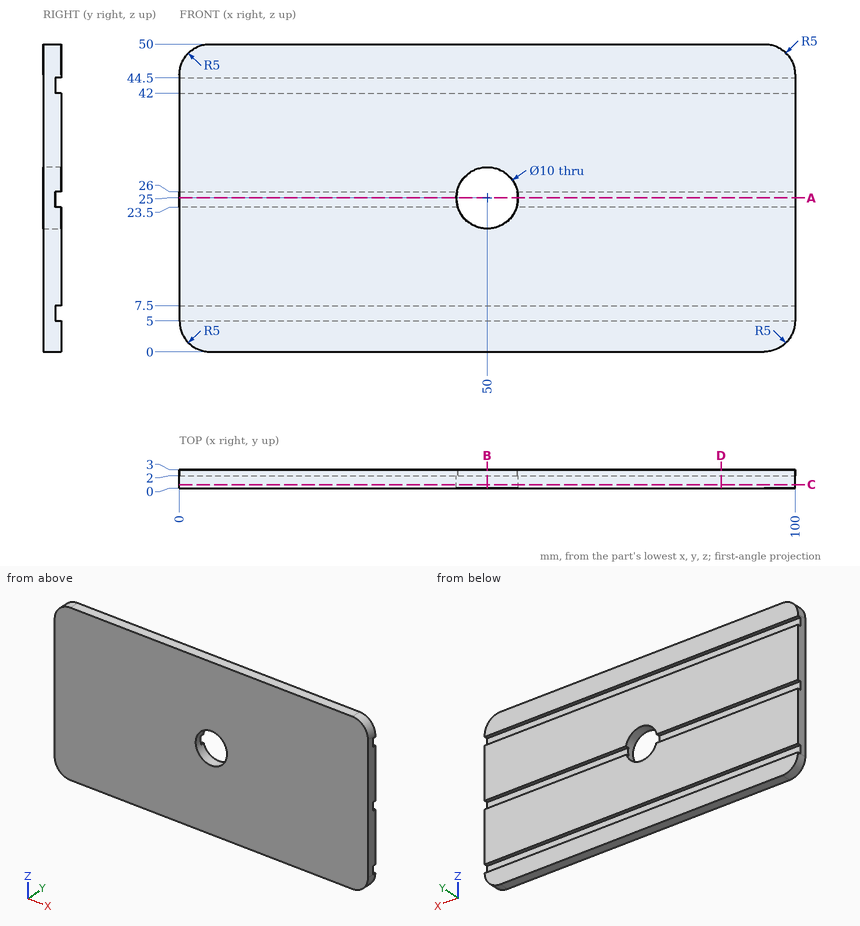
Part print with two shaded views. Sizes in mm from the minimum x, y, z corner. Round coordinates to 2 decimals unless told otherwise and drop trailing zeros. Order: outer loops, then holes, each group sorted by start corner. A loop starts at its lowest first (then second) coordinate and runs counter-clockwise, first axis right, second up. Notation, with made-up numbers: M -34,39 L -5,39 A33 ccw -5,73 Z; hole C 41,2.25 d5. An arc over 180 degrees is marked long. Use CSV: the item, a comma, the result in double quotes. Start each with the question number.
(1) Cut at D-D on x = 88. List the corners of the cut face in (y, z), then the cut area to 4 significant figures.
(2) Flat gauge pin, fed straight in: P1, Ø1.2, axis at x = 30, z = 6.5, coming from the +Y side. Where does the tip first touch, or does it go through?
(3) Drill centre lines: probe 1 along Z at (x, y) = (72, 2.55); probe 2 along Z at (x, y) = (50, 0.75); probe 3 along Z at (x, y) = (47, 2.7). Where is each one in solid material? Low to high.
(4) Cut at C-C on y = 0.6. List the corners of the cut face in (x, z).
(5) Cut at A-A on z = 25. List the corners of the cut face in (x, y).
(6) Cut at B-B on x = 50. List the corners of the cut face in (y, z), then the cut area to 3 significant figures.
Findings:
1,outline,"M 0,0 L 3,0 L 3,5 L 2,5 L 2,7.5 L 3,7.5 L 3,23.5 L 2,23.5 L 2,26 L 3,26 L 3,42 L 2,42 L 2,44.5 L 3,44.5 L 3,50 L 0,50 Z"
1,area,"142.5 mm^2"
2,P1,"stops at y = 2"
3,probe 1,"z = 0 to 5, 7.5 to 23.5, 26 to 42, 44.5 to 50"
3,probe 2,"z = 0 to 20, 30 to 50"
3,probe 3,"z = 0 to 5, 7.5 to 21, 29 to 42, 44.5 to 50"
4,outline,"M 0,5 A5 ccw 5,0 L 95,0 A5 ccw 100,5 L 100,45 A5 ccw 95,50 L 5,50 A5 ccw 0,45 Z; hole C 50,25 d10"
5,outline,"M 0,0 L 45,0 L 45,2 L 0,2 Z; M 55,0 L 100,0 L 100,2 L 55,2 Z"
6,outline,"M 0,0 L 3,0 L 3,5 L 2,5 L 2,7.5 L 3,7.5 L 3,20 L 0,20 Z; M 0,30 L 3,30 L 3,42 L 2,42 L 2,44.5 L 3,44.5 L 3,50 L 0,50 Z"
6,area,"115 mm^2"
